Check sheet for the drawn part. Datum: minimum x, y, z corner. Units: mm. Coordinates: 2 decimals unless noted, no trailing zeros. Write each loop counter-clockwise with the first axis right and the second up, starting at its lowest first coordinate (ties: lowest second). Pieces come first, ordered by that corner, then holes. Notation, with made-up numbers: (-31, -40) -> (3, -40) arc R27 ccw to (3, -2) -> close; hole circle Ø9 at (-30, 88.25). An arc over 180 degrees is marked (long way). Write each question's results on one line, items separated by ' | '. Start each with the question number.
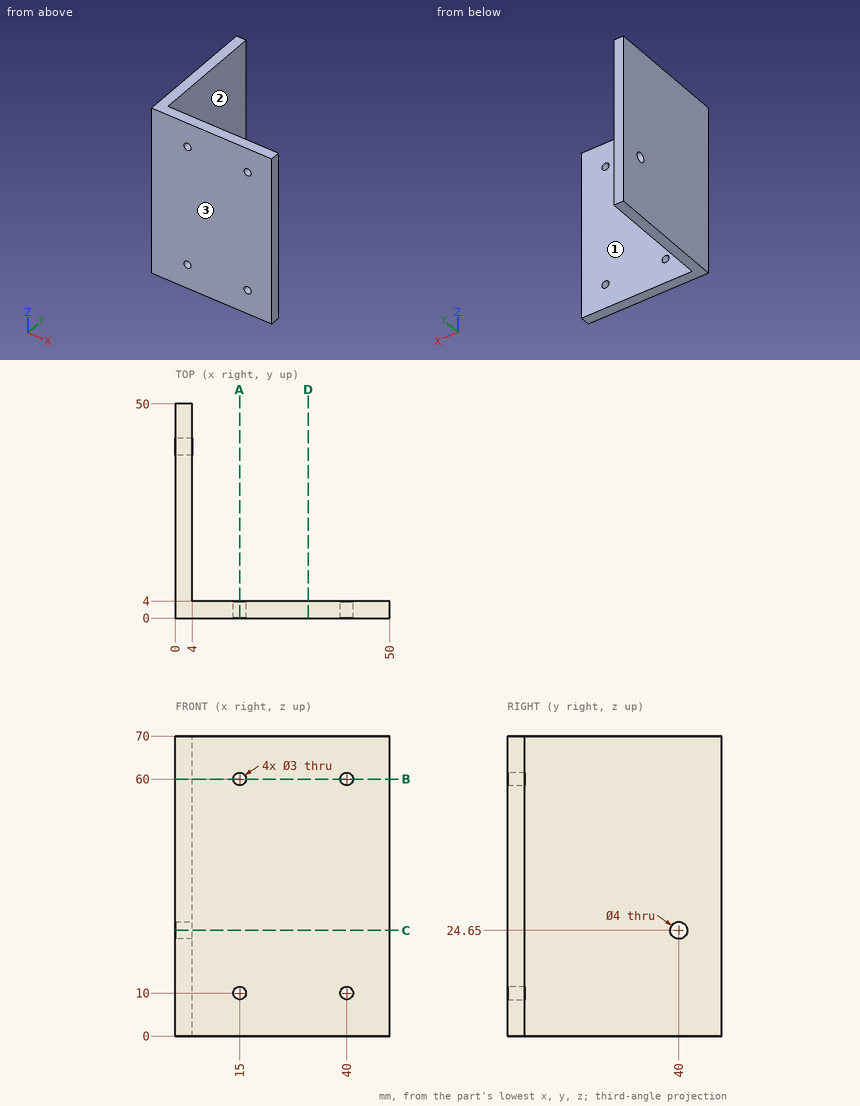
1. Depth check by flat-ended pin: pin 1 Ø1 at (x, z) = (9.5, 45) entering from +Y; pin 2 Ø1.5 at (y, z) = (31, 19) entering from +X; pin 3 Ø5 at (x, z) = (30, 61.5) entering from -Y. Enter the tip coordinate at first touch or a pass-through.
2. Sectioned sample at B-B on z = 60. Record the cut outline in (x, y).
3. Sectioned sample at D-D on x = 31. Record the cut outline in (y, z).
4. Sectioned sample at A-A on x = 15. Record the cut outline in (y, z).
5. Material ranges on probe 1 along X at (y, z) = (2, 10); probe 2 along Y at (x, z) = (1.05, 24.65); probe 3 along X at (y, z) = (38.5, 49.5), recorded low to high. Write a range as from..to.
6. Sectioned sample at C-C on z = 24.65. Record the cut outline in (x, y), plus the area to 3 significant figures.
7. Mould release check, pull along Y, two halves, no side actions. Record for the marked faces 1, 2 and 3: +Y half, -Y half, draft (parallel to the pull), parting line (faces both ways), or undercut.
Computed values:
1) pin 1: stops at y = 4 | pin 2: stops at x = 4 | pin 3: stops at y = 0
2) outline: (0, 0) -> (13.5, 0) -> (13.5, 4) -> (4, 4) -> (4, 50) -> (0, 50) -> close; (16.5, 0) -> (38.5, 0) -> (38.5, 4) -> (16.5, 4) -> close; (41.5, 0) -> (50, 0) -> (50, 4) -> (41.5, 4) -> close
3) outline: (0, 0) -> (4, 0) -> (4, 70) -> (0, 70) -> close
4) outline: (0, 0) -> (4, 0) -> (4, 8.5) -> (0, 8.5) -> close; (0, 11.5) -> (4, 11.5) -> (4, 58.5) -> (0, 58.5) -> close; (0, 61.5) -> (4, 61.5) -> (4, 70) -> (0, 70) -> close
5) probe 1: x = 0..13.5, 16.5..38.5, 41.5..50 | probe 2: y = 0..38, 42..50 | probe 3: x = 0..4
6) outline: (0, 0) -> (50, 0) -> (50, 4) -> (4, 4) -> (4, 38) -> (0, 38) -> close; (0, 42) -> (4, 42) -> (4, 50) -> (0, 50) -> close | area: 368 mm^2
7) face 1: +Y half | face 2: draft | face 3: -Y half
